from build123d import *

# Parameters (mm, degrees)
EXTRUDE_1_DEPTH         = 12
HOLE_WIZARD_M12_2_D     = 10.2
HOLE_WIZARD_M12_2_DEPTH = 32.75
HOLE_WIZARD_M12_2_TIP   = 3.064389157
FILLET_2_R              = 8


with BuildPart() as part:
    # 草图1 → 凸台-拉伸1 (new body)
    with BuildSketch(Plane.XY):
        with BuildLine():
            Line((-30.5, 61), (30.5, 61))
            Line((30.5, 61), (30.5, 0))
            Line((30.5, 0), (51.23475383, 0))
            ThreePointArc((51.23475383, 0), (65, 40), (51.23475383, 80))
            Line((51.23475383, 80), (0, 80))
            Line((0, 80), (-51.23475383, 80))
            ThreePointArc((-51.23475383, 80), (-65, 40), (-51.23475383, 0))
            Line((-51.23475383, 0), (-30.5, 0))
            Line((-30.5, 0), (-30.5, 61))
        make_face()
    extrude(amount=EXTRUDE_1_DEPTH)

    # M12 螺纹孔2
    with Locations(Plane.XY.offset(12)):
        with Locations((-50, 40), (50, 40)):
            Hole(HOLE_WIZARD_M12_2_D / 2, depth=HOLE_WIZARD_M12_2_DEPTH)
            with Locations((0, 0, -(HOLE_WIZARD_M12_2_DEPTH + HOLE_WIZARD_M12_2_TIP / 2))):  # 118° drill point
                Cone(0, HOLE_WIZARD_M12_2_D / 2, HOLE_WIZARD_M12_2_TIP, mode=Mode.SUBTRACT)

    # 圆角2
    fillet_2_edges = [part.edges().sort_by_distance(p)[0] for p in [
        (30.5, 61, 6),
        (-30.5, 61, 6),
    ]]
    fillet(fillet_2_edges, radius=FILLET_2_R)


solid = part.part
The listing builds one solid part. Answer for the finished solid, in the listing's coordinates (mm). A direction names the side the tool comes from. Coordinates: 2 decimals unless noted, no trailing zeros. Order: outer loops, then holes, each group sorted by start corner. A loop starts at its lowest first (then second) coordinate and runs counter-clockwise, first axis right, second up.
Q1. A cutting plane is placed at B-B, the plane y = 40. Write down the section's boundary in (x, z).
Q2. A cutting plane is placed at D-D, the plane y = 15.5. Write down the section's boundary in (x, z), and give its area (3 significant figures).
Q3. Consider line 1 (Y direction, x = 50, z = 8.25); line 2 (Y direction, x = -9.5, z = 7.5); line 3 (X direction, y = 55.5, z = 3.5). Determine where each line is inside the solid, lowest interval first.
Q4. Which of the six approach directions +Z, -Z, +X, -X, +Y, -Y give full straight-line access (tool end or side, diameter ignored) to faces 5 (the face through (1, 80, 6)), 6 (the face through (0, 61, 6))?
Q5. A cutting plane is placed at A-A, the plane x = 50. Write down the section's boundary in (y, z).
Q6. For a pull along Y with two mould halves and no side action, classify faces 1 (the face through (-1, 67, 12)), 2 (the face through (54.05, 36.9, 5.92)), 3 (the face through (64.997, 39.397, 5.916)), 4 (the face through (41, 0, 6)) as pulls with the +Y half, pulls with the -Y half, needs draft (parallel to the pull), parting line crosses it, or undercut.
Q7. A cutting plane is placed at C-C, the plane z = 3.5. Write down the section's boundary in (x, y), and give its area (3 significant figures).
Q8. Given P1, Ø1, axis at x = 9.5, z = 5, coming from the -Y side; P2, Ø6, axis at y = 21.5, z = 7.5, coming from the +X side; P3, Ø9, axis at x = -50, y = 40, coming from the +Z side; P4, Ø3, axis at y = 24.5, z = 7, coming from the -X side, each flat-ended and moving along its own axis, determine where each tip first touches the part or whether it passes through.
Answers follow:
1. outline: (-65, 0) - (-55.1, 0) - (-55.1, 12) - (-65, 12) - close; (-44.9, 0) - (-30.5, 0) - (-30.5, 12) - (-44.9, 12) - close; (30.5, 0) - (44.9, 0) - (44.9, 12) - (30.5, 12) - close; (55.1, 0) - (65, 0) - (65, 12) - (55.1, 12) - close
2. outline: (-60.21, 0) - (-30.5, 0) - (-30.5, 12) - (-60.21, 12) - close; (30.5, 0) - (60.21, 0) - (60.21, 12) - (30.5, 12) - close
2. area: 713 mm2
3. line 1: y = 0 to 34.9, 45.1 to 80
3. line 2: y = 61 to 80
3. line 3: x = -63.12 to -30.1, 30.1 to 63.12
4. face 5: +Z, -Z, +X, -X, +Y
4. face 6: +Z, -Z, -Y
5. outline: (0, 0) - (34.9, 0) - (34.9, 12) - (0, 12) - close; (45.1, 0) - (80, 0) - (80, 12) - (45.1, 12) - close
6. face 1: needs draft
6. face 2: undercut
6. face 3: parting line crosses it
6. face 4: pulls with the -Y half
7. outline: (-51.23, 0) - (-30.5, 0) - (-30.5, 53) arc R8 cw to (-22.5, 61) - (22.5, 61) arc R8 cw to (30.5, 53) - (30.5, 0) - (51.23, 0) arc R65 ccw to (51.23, 80) - (-51.23, 80) arc R65 ccw to start; hole circle Ø10.2 at (-50, 40); hole circle Ø10.2 at (50, 40)
7. area: 5,840 mm2
8. P1: stops at y = 61
8. P2: stops at x = 63.12
8. P3: passes through
8. P4: stops at x = -63.47
